```python
from build123d import *

# Parameters (mm, degrees)
F0_W     = 44.45
F0_H     = 107.95
F1_DEPTH = 12.7
F2_W     = 44.45
F2_H     = 12.7
F3_DEPTH = 38.1
F4_R     = 3.175
F5_DEPTH = 12.701


with BuildPart() as f1:
    # F0 (on Top) → F1 (new body)
    with BuildSketch(Plane.XY):
        with Locations((22.225, 53.975)):
            Rectangle(F0_W, F0_H)
    extrude(amount=F1_DEPTH)

    # F2 (on face) → F3 (join)
    with BuildSketch(Plane(origin=(0, 0, 0), x_dir=(1, 0, 0), z_dir=(0, 0, -1))):
        with Locations((22.225, -6.35)):
            Rectangle(F2_W, F2_H)
    extrude(amount=F3_DEPTH)

    # F4 (on face) → F5 (cut, through all)
    with BuildSketch(Plane(origin=(0, 12.7, 0), x_dir=(-1, 0, 0), z_dir=(0, 1, 0))):
        with Locations((-34.29, -10.16)):
            Circle(F4_R)
        with Locations((-34.29, -27.94)):
            Circle(F4_R)
        with Locations((-10.16, -10.16)):
            Circle(F4_R)
        with Locations((-10.16, -27.94)):
            Circle(F4_R)
    extrude(amount=-F5_DEPTH, mode=Mode.SUBTRACT)


solid = f1.part
```
Input: part model. Units: mm. Frame: model coordinates. A direction names the side the tool comes from. Round coordinates to 2 decimals unless told otherwise and drop trailing zeros. Loops run counter-clockwise (first coordinate to the right, second up) from the corner with the lowest first, then second, coordinate; pieces in that order, holes last. Notation, with made-up numbers: (57.25, 20.25) -> (80.25, 20.25) arc R29 ccw to (80.25, 50.25) -> close; hole circle Ø2 at (68.5, 52). An arc over 180 degrees is marked (long way). Write each question's results on one line, items separated by ' | '.
1. Section B-B (z = -10.16). Return loops of the section in (x, y) (3 decimals), and give its area (3 significant figures).
Geometry results:
outline: (0, 0) -> (6.985, 0) -> (6.985, 12.7) -> (0, 12.7) -> close; (13.335, 0) -> (31.115, 0) -> (31.115, 12.7) -> (13.335, 12.7) -> close; (37.465, 0) -> (44.45, 0) -> (44.45, 12.7) -> (37.465, 12.7) -> close | area: 403 mm2
2. Mould query, pull axis X, two halves, no side actions, for faces 3 (the face through (0, 46, 1)), 4 (the face through (8.695, 6.439, -12.977)), 5 (the face through (44.45, 46, 1)). Classes: +X half, -X half, draft (parallel to the pull), parting line (faces both ways), or undercut.
Geometry results:
face 3: -X half | face 4: undercut | face 5: +X half
3. Set-up query: faces 1 (the face through (22, 61, 0)), 2 (the face through (31.36, 6.44, -11.38)). Return all of +Z, -Z, +X, -X, +Y, -Y with unobstructed straight access to the full face (end or side cutting, diameter ignored); none if empty.
Geometry results:
face 1: -Z, +X, -X, +Y | face 2: +Y, -Y
4. Ray query, line 1 (Z direction, x = 34.29, y = 3.75) (3 decimals); line 2 (X direction, y = 5, z = -10); line 3 (X direction, y = 6, z = -27). Return the intervals inside material, ascending. Write a range as from..to.
Geometry results:
line 1: -38.1..-31.115, -24.765..-13.335, -6.985..12.7 | line 2: 0..6.99, 13.33..31.12, 37.46..44.45 | line 3: 0..7.13, 13.19..31.26, 37.32..44.45
5. Section C-C (y = 8). Return loops of the section in (x, z) (3 decimals), and give its area (3 significant figures).
Geometry results:
outline: (0, -38.1) -> (44.45, -38.1) -> (44.45, 12.7) -> (0, 12.7) -> close; hole circle Ø6.35 at (10.16, -27.94); hole circle Ø6.35 at (10.16, -10.16); hole circle Ø6.35 at (34.29, -27.94); hole circle Ø6.35 at (34.29, -10.16) | area: 2,130 mm2
6. First-contact query: P1, Ø8.5, axis at x = 34.29, z = -27.94, coming from the +Y side; P2, Ø6, axis at x = 7, y = 81.5, coming from the -Z side; P3, Ø8, axis at x = 28, z = -17.5, coming from the -Y side; P4, Ø5, axis at x = 10.16, z = -27.94, coming from the -Y side. Flat tips, straight axial feed; report the tip coordinate or a pass-through.
Geometry results:
P1: y = 12.7 | P2: z = 0 | P3: y = 0 | P4: through
7. Section A-A (x = 10.16). Return loops of the section in (y, z) (3 decimals).
Geometry results:
outline: (0, -38.1) -> (12.7, -38.1) -> (12.7, -31.115) -> (0, -31.115) -> close; (0, -24.765) -> (12.7, -24.765) -> (12.7, -13.335) -> (0, -13.335) -> close; (0, -6.985) -> (12.7, -6.985) -> (12.7, 0) -> (107.95, 0) -> (107.95, 12.7) -> (0, 12.7) -> close
8. Section D-D (x = 20). Return loops of the section in (y, z).
Geometry results:
outline: (0, -38.1) -> (12.7, -38.1) -> (12.7, 0) -> (107.95, 0) -> (107.95, 12.7) -> (0, 12.7) -> close
